from build123d import *
from build123d.topology import SkipClean


with BuildPart() as part:
    # Esquisse2 → R_volution1 (revolve)
    with BuildSketch(Plane.XY, mode=Mode.PRIVATE) as r_volution1_sk:
        with BuildLine():
            add(Edge.make_bspline(
                [(-0.25, 5.05698061), (-2.107045179, 5.402904177), (-0.86139121, 3.236013516), (-0.979154643, 2.5)],
                knots=[0.040200469, 0.040200469, 0.040200469, 0.040200469, 1, 1, 1, 1], degree=3))
            Line((-0.979154643, 2.5), (0, 2.5))
            Line((0, 2.5), (0, 5))
            Line((0, 5), (-0.25, 5))
            Line((-0.25, 5), (-0.25, 5.05698061))
        make_face()
        with BuildLine():
            Line((0, 2.5), (-0.979154643, 2.5))
            add(Edge.make_bspline(
                [(-0.25, -0.05698061), (-2.107045179, -0.402904177), (-0.86139121, 1.763986484), (-0.979154643, 2.5)],
                knots=[0.040200469, 0.040200469, 0.040200469, 0.040200469, 1, 1, 1, 1], degree=3))
            Line((-0.25, -0.05698061), (-0.25, 0))
            Line((-0.25, 0), (0, 0))
            Line((0, 0), (0, 2.5))
        make_face()
        with BuildLine():
            add(Edge.make_bspline(
                [(0, 0), (-0.088995136, -0.02359492), (-0.172219084, -0.042491867), (-0.25, -0.05698061)],
                knots=[0, 0, 0, 0, 0.040200469, 0.040200469, 0.040200469, 0.040200469], degree=3))
            Line((-0.25, -0.05698061), (-0.25, -1.25))
            Line((-0.25, -1.25), (0, -1.25))
            Line((0, -1.25), (0, 0))
        make_face()
        with BuildLine():
            Line((-0.25, 0), (-0.25, -0.05698061))
            add(Edge.make_bspline(
                [(0, 0), (-0.088995136, -0.02359492), (-0.172219084, -0.042491867), (-0.25, -0.05698061)],
                knots=[0, 0, 0, 0, 0.040200469, 0.040200469, 0.040200469, 0.040200469], degree=3))
            Line((0, 0), (-0.25, 0))
        make_face()
        with BuildLine():
            add(Edge.make_bspline(
                [(0, 5), (-0.088995136, 5.02359492), (-0.172219084, 5.042491867), (-0.25, 5.05698061)],
                knots=[0, 0, 0, 0, 0.040200469, 0.040200469, 0.040200469, 0.040200469], degree=3))
            Line((-0.25, 5.05698061), (-0.25, 5))
            Line((-0.25, 5), (0, 5))
        make_face()
        with BuildLine():
            Line((-0.25, 6.25), (-0.25, 5.05698061))
            add(Edge.make_bspline(
                [(0, 5), (-0.088995136, 5.02359492), (-0.172219084, 5.042491867), (-0.25, 5.05698061)],
                knots=[0, 0, 0, 0, 0.040200469, 0.040200469, 0.040200469, 0.040200469], degree=3))
            Line((0, 5), (0, 6.25))
            Line((0, 6.25), (-0.25, 6.25))
        make_face()
    revolve(r_volution1_sk.sketch.rotate(Axis((0, 0, 0), (0, 1, 0)), 270), axis=Axis((0, 0, 0), (0, 1, 0)))

    # Esquisse4 → R_volution2 (revolve)
    with SkipClean():  # the faces are left unmerged after this step: merging them gives an invalid solid
        with BuildSketch(Plane(origin=(0, -1.25, 0), x_dir=(-1, 0, 0), z_dir=(0, -1, 0)), mode=Mode.PRIVATE) as r_volution2_sk:
            with BuildLine():
                Line((0, -4), (0, -0.25))
                ThreePointArc((0, -0.25), (-0.176776695, -0.176776695), (-0.25, 0))
                Line((-0.25, 0), (-0.25, -4))
                Line((-0.25, -4), (0, -4))
            make_face()
            with BuildLine():
                ThreePointArc((0.25, 0), (0.176776695, 0.176776695), (0, 0.25))
                Line((0, 0.25), (0, -0.25))
                ThreePointArc((0, -0.25), (0.176776695, -0.176776695), (0.25, 0))
            make_face()
            with BuildLine():
                Line((0, -0.25), (0, 0.25))
                ThreePointArc((0, 0.25), (-0.176776695, 0.176776695), (-0.25, 0))
                ThreePointArc((-0.25, 0), (-0.176776695, -0.176776695), (0, -0.25))
            make_face()
        revolve(r_volution2_sk.sketch.rotate(Axis((0, -1.25, 0), (0, 0, 1)), 180), axis=Axis((0, -1.25, 0), (0, 0, 1)))
    add(part.part.scale(1), mode=Mode.REPLACE)  # the faces are merged on a copy

    # Esquisse5 → R_volution3 (revolve)
    with BuildSketch(Plane(origin=(0, 6.25, 0), x_dir=(1, 0, 0), z_dir=(0, 1, 0))):
        with BuildLine():
            ThreePointArc((0, -0.25), (-0.176776695, -0.176776695), (-0.25, 0))
            Line((-0.25, 0), (-0.25, -4))
            Line((-0.25, -4), (0, -4))
            Line((0, -4), (0, -0.25))
        make_face()
        with BuildLine():
            Line((0, -0.25), (0, 0))
            Line((0, 0), (-0.25, 0))
            ThreePointArc((-0.25, 0), (-0.176776695, -0.176776695), (0, -0.25))
        make_face()
        with BuildLine():
            Line((-0.25, 0), (0, 0))
            Line((0, 0), (0, 0.25))
            ThreePointArc((0, 0.25), (-0.176776695, 0.176776695), (-0.25, 0))
        make_face()
    revolve(axis=Axis((0, 6.25, 0), (0, 0, 1)))


solid = part.part
Input: part model. Units: mm. Frame: model coordinates. Coordinates: 2 decimals unless noted, no trailing zeros. Order: outer loops, then holes, each group sorted by start corner. A loop starts at its lowest first (then second) coordinate and runs counter-clockwise, first axis right, second up. Notation, with made-up numbers: M 86.5,39 L 108.5,39 A16 cw 108.5,63 Z; hole C -14.5,55.25 d8. An arc over 180 degrees is marked long. One line per question, with ' | ' between items.
Item 1: Pin query (flat end, axial travel): pin 1 (1.5 mm diameter, centred on y = 1.5, z = 0, fed in from -X). Return the tip coordinate at first contact, or that it passes through.
Geometry results:
pin 1: stops at x = -1.27
Item 2: Section A-A (z = 3.05). Output: boundary loops of the cut face in (x, y).
Geometry results:
outline: C 0,-1.25 d0.5; C 0,6.25 d0.5
Item 3: Ray query, line 1 along Z through (x, y) = (-0.15, 4); line 2 along Z through (x, y) = (0.4, 1.25); line 3 along Y through (x, z) = (-0.45, -0.7). Return the intervals inside material, ascending.
Geometry results:
line 1: z = -1.23 to 1.23 | line 2: z = -1.12 to 1.12 | line 3: y = -0.07 to 5.07
